Model file for the job. Use its own axes, mm. Face numbers are marked on the shaded views. A direction names the side the tool comes from. Round coordinates to 2 decimals unless told otherwise and drop trailing zeros. Order: outer loops, then holes, each group sorted by start corner. A loop starts at its lowest first (then second) coordinate and runs counter-clockwise, first axis right, second up. Notation, with made-up numbers: (58.5, 77) - (81.5, 77) arc R9 ccw to (81.5, 81) - close; hole circle Ø9 at (27.25, -2). An arc over 180 degrees is marked (long way). Write item = value, one per line. Start each with the question number.
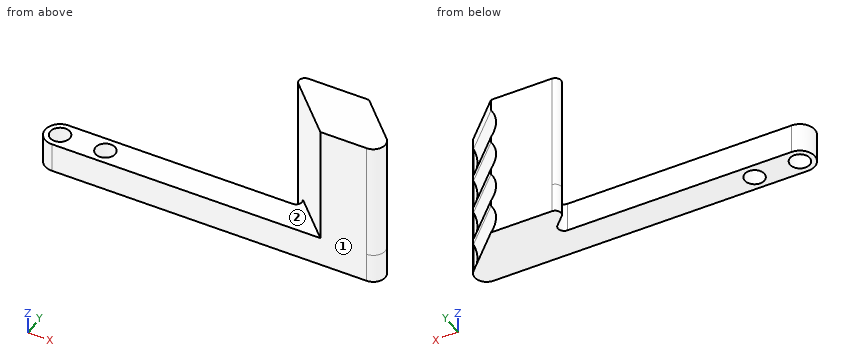
from build123d import *

# Parameters (mm, degrees)
SKETCH2_R           = 1.65
BOSS_EXTRUDE1_DEPTH = 5
FILLET1_R           = 2
FILLET2_R           = 1
FILLET3_R           = 1
SKETCH3_R           = 5.5
CUT_EXTRUDE1_DEPTH  = 34
BOSS_EXTRUDE2_DEPTH = 20
LPATTERN1_COUNT     = 4
LPATTERN1_PITCH     = 6


with BuildPart() as part:
    # Sketch2 → Boss-Extrude1 (new body)
    with BuildSketch(Plane.XY):
        with BuildLine():
            Line((40, 2.5), (0, 2.5))
            ThreePointArc((0, 2.5), (-2.5, 0), (0, -2.5))
            Line((0, -2.5), (57.6, -2.5))
            Line((57.6, -2.5), (47.6, 7.5))
            Line((47.6, 7.5), (35, 7.5))
            Line((35, 7.5), (40, 2.5))
        make_face()
        with Locations((7.6, 0)):
            Circle(SKETCH2_R, mode=Mode.SUBTRACT)
        Circle(SKETCH2_R, mode=Mode.SUBTRACT)
    extrude(amount=BOSS_EXTRUDE1_DEPTH)

    # Fillet1
    fillet1_edges = [part.edges().sort_by_distance(p)[0] for p in [
        (57.6, -2.5, 2.5),
    ]]
    fillet(fillet1_edges, radius=FILLET1_R)

    # Fillet2
    fillet2_edges = [part.edges().sort_by_distance(p)[0] for p in [
        (40, 2.5, 2.5),
    ]]
    fillet(fillet2_edges, radius=FILLET2_R)

    # Fillet3
    fillet3_edges = [part.edges().sort_by_distance(p)[0] for p in [
        (35, 7.5, 2.5),
    ]]
    fillet(fillet3_edges, radius=FILLET3_R)

    # Sketch3 → Cut-Extrude1 (cut)
    with BuildSketch(Plane(origin=(26.635786438, -26.635786438, 0), x_dir=(0, 0, -1), z_dir=(0.707106781, -0.707106781, 0))):
        with Locations((-2.5, 43.860563129)):
            Circle(SKETCH3_R)
    cut_extrude1 = extrude(amount=-CUT_EXTRUDE1_DEPTH, mode=Mode.SUBTRACT)

    # Sketch4 → Boss-Extrude2 (add)
    with BuildSketch(Plane.XY.offset(5)):
        with BuildLine():
            Line((37.414213562, 7.5), (47.6, 7.5))
            Line((47.6, 7.5), (54.185786438, 0.914213562))
            ThreePointArc((54.185786438, 0.914213562), (54.61933194, -1.265366865), (52.771572875, -2.5))
            Line((52.771572875, -2.5), (45, -2.5))
            Line((45, -2.5), (38.292893219, 4.207106781))
            Line((38.292893219, 4.207106781), (36.707106781, 5.792893219))
            ThreePointArc((36.707106781, 5.792893219), (36.49033403, 6.882683432), (37.414213562, 7.5))
        make_face()
    extrude(amount=BOSS_EXTRUDE2_DEPTH)

    # LPattern1: Cut-Extrude1 ×4
    with Locations(*[(0, 0, i * LPATTERN1_PITCH) for i in range(1, LPATTERN1_COUNT)]):
        add(cut_extrude1, mode=Mode.SUBTRACT)


solid = part.part
Item 1: Saw through at C-C, the plane x = 40.5. Give the cut face in (y, z).
Item 2: Probe L1, parallel to Y at x = 7.6, z = 3.25; L2, parallel to Y at x = 42, z = 19.75; L3, parallel to Z at x = 5.5, y = -0.75. List the from-to ranges inside material, lowest first.
Item 3: Saw through at B-B, the plane z = 3.75. Give the cut face in (x, y), then the cut area to 3 significant figures.
Item 4: Which spindle directions (+Z, -Z, +X, -X, +Y, -Y) get a long thin tool onto all of the face, cutting with end or side? Do the marked faces 1 and 2. Say none if no direction does.
Item 5: Saw through at D-D, the plane z = 9.5. Give the cut face in (x, y), then the cut area to 3 significant figures.
Item 6: Saw through at A-A, the plane x = 7.6. Give the cut face in (y, z).
Item 7: Drop flat-ended pins along their axis: pin 1 (1.5 mm diameter, centred on y = 5, z = 19.5, fed in from -X); pin 2 (5 mm diameter, centred on x = 35.5, y = 2, fed in from +Z); pin 3 (4 mm diameter, centred on x = 12.5, z = 2.5, fed in from +Y); pin 4 (2.5 mm diameter, centred on x = 0, y = 0, fed in from -Z). Give the stop position or say it passes through.
Check sheet entries:
q1.outline = (-2.5, 0) - (7.5, 0) - (7.5, 25) - (2, 25) - (2, 5) - (-2.5, 5) - close
q2.L1 = -2.5 to -1.65, 1.65 to 2.5
q2.L2 = 0.5 to 7.5
q2.L3 = 0 to 5
q3.outline = (0, -2.5) - (52.77, -2.5) arc R2 ccw to (54.19, 0.91) - (53.86, 0.59) - (46.95, 7.5) - (37.41, 7.5) arc R1 ccw to (36.71, 5.79) - (38.29, 4.21) arc R1 cw to (37.59, 2.5) - (0, 2.5) arc R2.5 ccw to start; hole circle Ø3.3 at (0, 0); hole circle Ø3.3 at (7.6, 0)
q3.area = 322 mm2
q4.face_1 = +Z, -Z, +X, -X, -Y
q4.face_2 = +Z, -X, -Y
q5.outline = (36.71, 5.79) - (45, -2.5) - (52.77, -2.5) arc R2 ccw to (54.19, 0.91) - (53.83, 0.55) - (46.88, 7.5) - (37.41, 7.5) arc R1 ccw to start
q5.area = 115 mm2
q6.outline = (-2.5, 0) - (-1.65, 0) - (-1.65, 5) - (-2.5, 5) - close; (1.65, 0) - (2.5, 0) - (2.5, 5) - (1.65, 5) - close
q7.pin_1 = 36.75
q7.pin_2 = 5
q7.pin_3 = 2.5
q7.pin_4 = through
